```python
from build123d import *

# Parameters (mm, degrees)
F0_R     = 25.4
F1_DEPTH = 355.6
F2_R     = 5.08
F3_R     = 5.08
F4_R     = 8.254169
F5_DEPTH = 88.9


with BuildPart() as f1:
    # F0 (on Front) → F1 (new body)
    with BuildSketch(Plane.XZ):
        Circle(F0_R)
    extrude(amount=F1_DEPTH)

    # F2
    f2_edges = [f1.edges().sort_by_distance(p)[0] for p in [
        (-25.4, -355.6, 0),
    ]]
    fillet(f2_edges, radius=F2_R)

    # F3
    f3_edges = [f1.edges().sort_by_distance(p)[0] for p in [
        (-25.4, 0, 0),
    ]]
    fillet(f3_edges, radius=F3_R)

    # F4 (on Top) → F5 (cut, symmetric)
    with BuildSketch(Plane.XY):
        with Locations((0, -151.942372)):
            Circle(F4_R)
    extrude(amount=F5_DEPTH, both=True, mode=Mode.SUBTRACT)


solid = f1.part
```
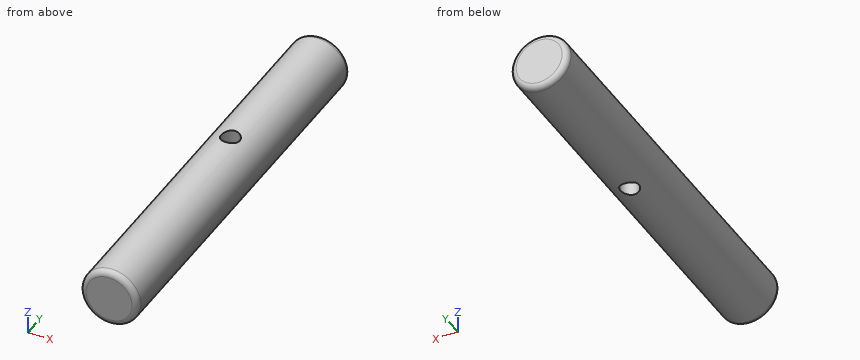
Read the model definition and answer for the solid it produces. Units are mm, in the model's axes. Round coordinates to 2 decimals unless told otherwise and drop trailing zeros. Write each loop counter-clockwise with the first axis right and the second up, starting at its lowest first coordinate (ties: lowest second). Pieces come first, ordered by that corner, then holes. Notation, with made-up numbers: (34.5, 16) -> (39.5, 16) arc R9 ccw to (39.5, 30) -> close; hole circle Ø7 at (69.25, 28). An arc over 180 degrees is marked (long way). Answer in a Markdown table with one row per item. Add a question column.
1) Consider line 1 (Y direction, x = 0, z = -4); line 2 (Y direction, x = -7, z = 3); line 3 (Y direction, x = 10, z = 18.5). Determine where each line is inside the solid, lowest interval first.
2) Find section B-B, the plane y = -42. Determine the outline of the cut face in (x, z), and give its area (3 significant figures).
3) Given P1, Ø3, axis at y = -98, z = 13.5, coming from the -X side; P2, Ø1, axis at y = -131.5, z = -2, coming from the +X side; P3, Ø5, axis at y = -165.5, z = 19, coming from the +X side, each flat-ended and moving along its own axis, determine where each tip first touches the part or whether it passes through.
4) Find section A-A, the plane x = 0. Determine the outline of the cut face in (y, z).
Findings below:
| question | item | result |
|---|---|---|
| 1 | line 1 | -355.6 to -160.2, -143.69 to 0 |
| 1 | line 2 | -355.6 to -156.32, -147.57 to 0 |
| 1 | line 3 | -355.55 to -0.05 |
| 2 | outline | circle Ø50.8 at (0, 0) |
| 2 | area | 2,030 mm² |
| 3 | P1 | x = -22.39 |
| 3 | P2 | x = 25.36 |
| 3 | P3 | x = 19.31 |
| 4 | outline | (-355.6, -20.32) arc R5.08 ccw to (-350.52, -25.4) -> (-160.2, -25.4) -> (-160.2, 25.4) -> (-350.52, 25.4) arc R5.08 ccw to (-355.6, 20.32) -> close; (-143.69, -25.4) -> (-5.08, -25.4) arc R5.08 ccw to (0, -20.32) -> (0, 20.32) arc R5.08 ccw to (-5.08, 25.4) -> (-143.69, 25.4) -> close |
